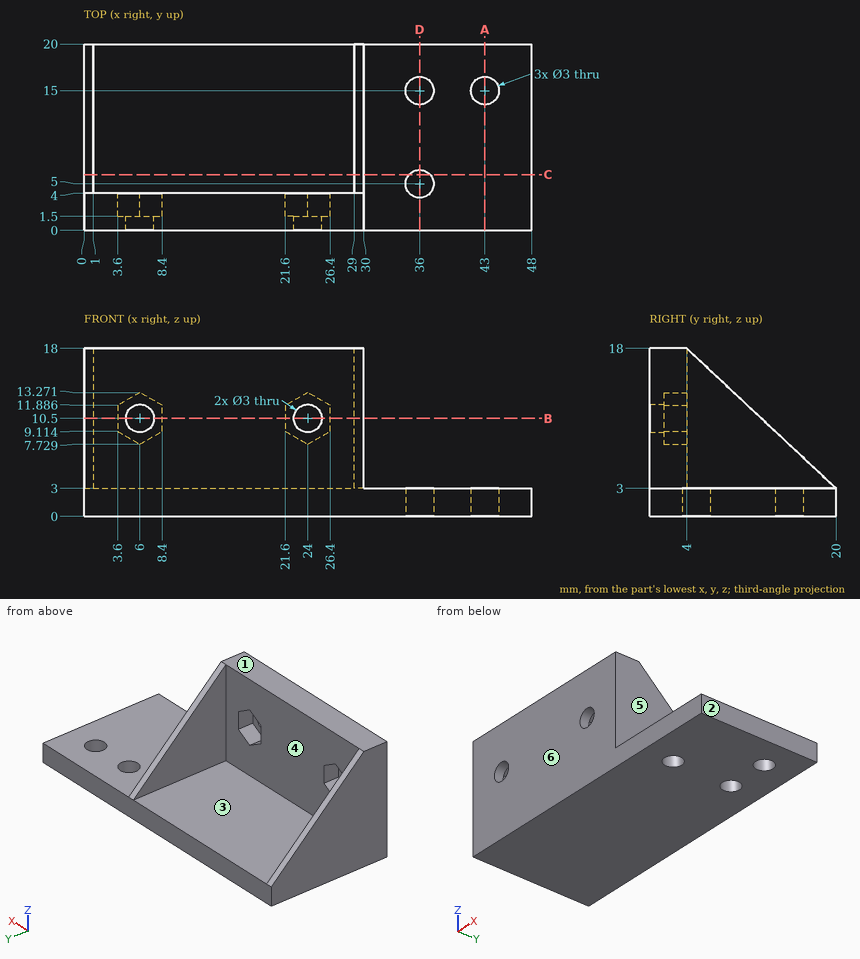
Job drawing, mm, ordinate dimensions from the low corner. One solid piece. A direction names the side the tool comes from. Coordinates: 2 decimals unless noted, no trailing zeros. Write each loop counter-clockwise with the first axis right and the second up, starting at its lowest first coordinate (ties: lowest second). Pieces come first, ordered by that corner, then holes. Notation, with made-up numbers: M 62,8.5 L 119,8.5 A35 cw 119,42.5 Z; hole C 57.5,21 d11. An arc over 180 degrees is marked long. Answer as a JSON object with one key per item and string values. Group by question number.
1) Pin check, flat tips, straight feed: pin 1 Ø4.5 at (y, z) = (11, 9) entering from +X; pin 2 Ø7.5 at (x, z) = (14.5, 12.5) entering from +Y; pin 3 Ø4 at (x, z) = (6, 10.5) entering from +Y. Stop position of each tip, or through.
2) Tool access for the marked faces 4, 5 and 6: list every direction of +Z, -Z, +X, -X, +Y, -Y with a clear straight run to the whole face (end or side of a thin tool).
3) Wall check: line 1 (Y direction, x = 36, z = 0.7); line 2 (Z direction, x = 24, y = 0.9); line 3 (X direction, y = 6.5, z = 8). Give the ranges that are in metal, low to high. Write a range as from..to.
4) Saw through at D-D (x = 36). Write the cut outline in (y, z).
5) Saw through at B-B (z = 10.5). Write the cut outline in (x, y), plus the area to 3 significant figures.
6) Saw through at A-A (x = 43). Write the cut outline in (y, z).
7) Mould opens along X. For the marked faces 1, 2 and 3 say: +X half, -X half, draft (parallel to the pull), parting line (faces both ways), or undercut.
8) Saw through at C-C (y = 6). Write the cut outline in (x, z) (1 decimal).
Values follow:
{
 "1": {"pin 1": "stops at x = 30", "pin 2": "stops at y = 4", "pin 3": "stops at y = 1.5"},
 "2": {"face 4": "+Z, +Y", "face 5": "+Z, +X, +Y, -Y", "face 6": "+Z, -Z, +X, -X, -Y"},
 "3": {"line 1": "y = 0..3.5, 6.5..13.5, 16.5..20", "line 2": "z = 0..9, 12..18", "line 3": "x = 0..1, 29..30"},
 "4": {"outline": "M 0,0 L 3.5,0 L 3.5,3 L 0,3 Z; M 6.5,0 L 13.5,0 L 13.5,3 L 6.5,3 Z; M 16.5,0 L 20,0 L 20,3 L 16.5,3 Z"},
 "5": {"outline": "M 0,0 L 4.5,0 L 4.5,1.5 L 3.6,1.5 L 3.6,4 L 1,4 L 1,12 L 0,12 Z; M 7.5,0 L 22.5,0 L 22.5,1.5 L 21.6,1.5 L 21.6,4 L 8.4,4 L 8.4,1.5 L 7.5,1.5 Z; M 25.5,0 L 30,0 L 30,12 L 29,12 L 29,4 L 26.4,4 L 26.4,1.5 L 25.5,1.5 Z", "area": "103 mm2"},
 "6": {"outline": "M 0,0 L 13.5,0 L 13.5,3 L 0,3 Z; M 16.5,0 L 20,0 L 20,3 L 16.5,3 Z"},
 "7": {"face 1": "draft", "face 2": "+X half", "face 3": "undercut"},
 "8": {"outline": "M 0,0 L 34.9,0 L 34.9,3 L 30,3 L 30,16.1 L 29,16.1 L 29,3 L 1,3 L 1,16.1 L 0,16.1 Z; M 37.1,0 L 48,0 L 48,3 L 37.1,3 Z"}
}
